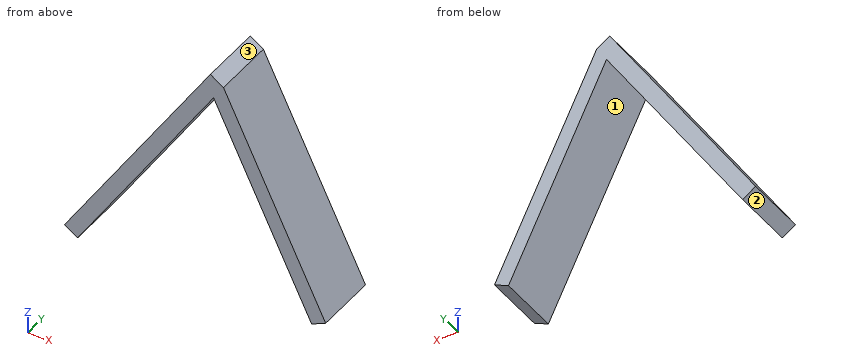
```python
from build123d import *

# Parameters (mm, degrees)
F1_E0_W  = 43.5960156369
F1_E0_H  = 10
F2_DEPTH = 2.54
F1_E1_W  = 37.7890589032
F1_E1_H  = 10
F3_DEPTH = 2.54


with BuildPart() as f2:
    # F1_E0 (on explicit) → F2 (new body)
    with BuildSketch(Plane(origin=(-52.6879653335, 0, -36.5696884692), x_dir=(0.5443919443, 0, 0.8388309788), z_dir=(0.8388309788, 0, -0.5443919443))):
        with Locations((21.7980078184, 5)):
            Rectangle(F1_E0_W, F1_E0_H)
    extrude(amount=-F2_DEPTH)

    # F1_E1 (on explicit) → F3 (join)
    with BuildSketch(Plane(origin=(-28.9546456188, 0, 0), x_dir=(0.4396331317, 0, -0.8981774376), z_dir=(-0.8981774376, 0, -0.4396331317))):
        with Locations((18.8945294516, 5)):
            Rectangle(F1_E1_W, F1_E1_H)
    extrude(amount=F3_DEPTH)


solid = f2.part
```
Geometry: final body of the model. Coordinates: model frame, mm. Face numbers are marked on the shaded views. Coordinates: 2 decimals unless noted, no trailing zeros. Order: outer loops, then holes, each group sorted by start corner. A loop starts at its lowest first (then second) coordinate and runs counter-clockwise, first axis right, second up. Notation, with made-up numbers: (79.5, -12) -> (87.5, -12) arc R4 cw to (87.5, -5) -> close; hole circle Ø5 at (-32.75, 49). An arc over 180 degrees is marked (long way). Use CSV: the item, a comma, the result in double quotes.
1) Mould query, pull axis X, two halves, no side actions, for the marked faces 1, 2 and 3. Classes: +X half, -X half, draft (parallel to the pull), parting line (faces both ways), or undercut.
Findings:
face 1,"undercut"
face 2,"-X half"
face 3,"+X half"
2) Section D-D on x = -30. Output: boundary loops of the cut face in (y, z).
Findings:
outline,"(-10, -3.64) -> (0, -3.64) -> (0, 0.68) -> (-10, 0.68) -> close"
3) Section C-C on x = -51.5. Output: boundary loops of the cut face in (y, z), then the cut area to 3 significant figures.
Findings:
outline,"(-10, -34.74) -> (0, -34.74) -> (0, -30.07) -> (-10, -30.07) -> close"
area,"46.7 mm^2"
4) Pin query (flat end, axial travel): pin 1 Ø1 at (y, z) = (-6.5, -26) entering from +X; pin 2 Ø5 at (y, z) = (-2, -6) entering from +X; pin 3 Ø1.5 at (y, z) = (-7, -26) entering from -X. Return the tip coordinate at first contact, or that it passes through.
Findings:
pin 1,"stops at x = -15.98"
pin 2,"stops at x = -24.79"
pin 3,"stops at x = -49.34"
5) Section B-B on z = -23.5. Output: boundary loops of the cut face in (x, y).
Findings:
outline,"(-47.23, -10) -> (-44.21, -10) -> (-44.21, 0) -> (-47.23, 0) -> close; (-20.28, -10) -> (-17.45, -10) -> (-17.45, 0) -> (-20.28, 0) -> close"
6) Section A-A on y = -5.25. Output: boundary loops of the cut face in (x, z), then the cut area to 3 significant figures.
Findings:
outline,"(-54.82, -35.19) -> (-52.69, -36.57) -> (-30.57, -2.48) -> (-14.62, -35.06) -> (-12.34, -33.94) -> (-28.95, 0) -> (-31.09, 1.38) -> close"
area,"205 mm^2"
7) Line query: line 1 (X direction, y = -2.5, z = -7); line 2 (X direction, y = -3, z = -11.5); line 3 (Z direction, x = -38, y = -6.5). Output: solid intervals per line, ascending.
Findings:
line 1,"x = -36.53 to -33.5, -28.36 to -25.53"
line 2,"x = -39.45 to -36.42, -26.15 to -23.33"
line 3,"z = -13.94 to -9.27"
